Here's how the part is built. I have some questions about the finished solid (model axes, mm). A direction names the side the tool comes from. Give positions to 0.01 mm unless a question says otherwise; leave off trailing zeros. Write each loop counter-clockwise with the first axis right and the second up, starting at its lowest first coordinate (ties: lowest second). Pieces come first, ordered by that corner, then holes. Notation, with made-up numbers: (31, 41.25) - (87, 41.25) arc R33 ccw to (87, 73.25) - close; hole circle Ø7 at (70, 9). An arc over 180 degrees is marked (long way). Use one line per item in the form item = value. Start each with the question number.
from build123d import *

# Parameters (mm, degrees)
SKETCH1_W           = 158.75
SKETCH1_H           = 390.525
BOSS_EXTRUDE1_DEPTH = 3.175
SKETCH2_W           = 101.6
SKETCH2_H           = 3.175
BOSS_EXTRUDE2_DEPTH = 3.175
SKETCH3_W           = 3.175
SKETCH3_H           = 101.6
BOSS_EXTRUDE3_DEPTH = 3.175
SKETCH4_R           = 1.5875
SKETCH4_R_2         = 57.5
CUT_EXTRUDE1_DEPTH  = 426.710554544
CUT_EXTRUDE2_DEPTH  = 426.710554544
FILLET1_R           = 1.5875
FILLET2_R           = 1.5875
SKETCH7_W           = 12.7
SKETCH7_H           = 12.7
CUT_EXTRUDE3_DEPTH  = 426.710554544


with BuildPart() as part:
    # Sketch1 → Boss-Extrude1 (new body)
    with BuildSketch(Plane(origin=(0, 0, 0), x_dir=(1, 0, 0), z_dir=(0, 1, 0))):
        with Locations((79.375, 195.2625)):
            Rectangle(SKETCH1_W, SKETCH1_H)
    extrude(amount=BOSS_EXTRUDE1_DEPTH)

    # Sketch2 → Boss-Extrude2 (add)
    with BuildSketch(Plane(origin=(0, 0, 0), x_dir=(1, 0, 0), z_dir=(0, 1, 0))):
        with Locations((79.375, 392.1125)):
            Rectangle(SKETCH2_W, SKETCH2_H)
        with Locations((79.375, -1.5875)):
            Rectangle(SKETCH2_W, SKETCH2_H)
    extrude(amount=BOSS_EXTRUDE2_DEPTH)

    # Sketch3 → Boss-Extrude3 (add)
    with BuildSketch(Plane(origin=(0, 0, 0), x_dir=(1, 0, 0), z_dir=(0, 1, 0))):
        with Locations((-1.5875, 296.8625)):
            Rectangle(SKETCH3_W, SKETCH3_H)
        with Locations((-1.5875, 93.6625)):
            Rectangle(SKETCH3_W, SKETCH3_H)
        with Locations((160.3375, 93.6625)):
            Rectangle(SKETCH3_W, SKETCH3_H)
        with Locations((160.3375, 296.8625)):
            Rectangle(SKETCH3_W, SKETCH3_H)
    extrude(amount=BOSS_EXTRUDE3_DEPTH)

    # Sketch4 → Cut-Extrude1 (cut, through all)
    with BuildSketch(Plane(origin=(0, 3.175, 0), x_dir=(1, 0, 0), z_dir=(0, 1, 0))):
        with Locations(Location((26.19375, 375.4374, 0), (0, 0, 270))):
            Circle(SKETCH4_R)
        with Locations(Location((132.55625, 375.4374, 0), (0, 0, 270))):
            Circle(SKETCH4_R)
        with Locations(Location((26.19375, 269.0749, 0), (0, 0, 270))):
            Circle(SKETCH4_R)
        with Locations(Location((132.55625, 269.0749, 0), (0, 0, 270))):
            Circle(SKETCH4_R)
        with Locations(Location((79.375, 322.25615, 0), (0, 0, 270))):
            Circle(SKETCH4_R_2)
    extrude(amount=-CUT_EXTRUDE1_DEPTH, mode=Mode.SUBTRACT)

    # Sketch5 → Cut-Extrude2 (cut, through all)
    with BuildSketch(Plane(origin=(0, 3.175, 0), x_dir=(1, 0, 0), z_dir=(0, 1, 0))):
        Polygon((71.75615, 243.20615), (19.05, 190.5), (19.05, 171.45), (90.80615, 243.20615), align=None)
        Polygon((109.85615, 243.20615), (19.05, 152.4), (19.05, 133.35), (128.90615, 243.20615), align=None)
        Polygon((139.7, 234.95), (19.05, 114.3), (19.05, 95.25), (139.7, 215.9), align=None)
        Polygon((139.7, 196.85), (19.05, 76.2), (19.05, 57.15), (139.7, 177.8), align=None)
        Polygon((139.7, 158.75), (19.05, 38.1), (19.05, 19.05), (139.7, 139.7), align=None)
        Polygon((139.7, 120.65), (38.1, 19.05), (57.15, 19.05), (139.7, 101.6), align=None)
        Polygon((139.7, 82.55), (76.2, 19.05), (95.25, 19.05), (139.7, 63.5), align=None)
        Polygon((139.7, 44.45), (114.3, 19.05), (133.35, 19.05), (139.7, 25.4), align=None)
    extrude(amount=-CUT_EXTRUDE2_DEPTH, mode=Mode.SUBTRACT)

    # Fillet1
    fillet1_edges = [part.edges().sort_by_distance(p)[0] for p in [
        (0, 1.5875, -347.6625),
        (-3.175, 1.5875, -347.6625),
        (-3.175, 1.5875, -246.0625),
        (0, 1.5875, -246.0625),
        (0, 1.5875, -144.4625),
        (-3.175, 1.5875, -144.4625),
        (-3.175, 1.5875, -42.8625),
        (0, 1.5875, -42.8625),
        (0, 1.5875, 0),
        (28.575, 1.5875, 0),
        (28.575, 1.5875, 3.175),
        (130.175, 1.5875, 3.175),
        (130.175, 1.5875, 0),
        (158.75, 1.5875, 0),
        (161.925, 1.5875, -42.8625),
        (158.75, 1.5875, -42.8625),
        (161.925, 1.5875, -144.4625),
        (158.75, 1.5875, -144.4625),
        (158.75, 1.5875, -246.0625),
        (161.925, 1.5875, -246.0625),
        (161.925, 1.5875, -347.6625),
        (158.75, 1.5875, -347.6625),
        (158.75, 1.5875, -390.525),
        (130.175, 1.5875, -390.525),
        (130.175, 1.5875, -393.7),
        (28.575, 1.5875, -393.7),
        (28.575, 1.5875, -390.525),
        (0, 1.5875, -390.525),
    ]]
    fillet(fillet1_edges, radius=FILLET1_R - 0.0001)  # a hair under: the kernel refuses the full size

    # Fillet2
    fillet2_edges = [part.edges().sort_by_distance(p)[0] for p in [
        (19.05, 1.5875, -38.1),
        (139.7, 1.5875, -158.75),
        (139.7, 1.5875, -139.7),
        (19.05, 1.5875, -19.05),
        (19.05, 1.5875, -76.2),
        (139.7, 1.5875, -196.85),
        (139.7, 1.5875, -177.8),
        (19.05, 1.5875, -57.15),
        (95.25, 1.5875, -19.05),
        (76.2, 1.5875, -19.05),
        (139.7, 1.5875, -82.55),
        (139.7, 1.5875, -63.5),
        (57.15, 1.5875, -19.05),
        (38.1, 1.5875, -19.05),
        (139.7, 1.5875, -120.65),
        (139.7, 1.5875, -101.6),
        (19.05, 1.5875, -190.5),
        (71.75615, 1.5875, -243.20615),
        (90.80615, 1.5875, -243.20615),
        (19.05, 1.5875, -171.45),
        (19.05, 1.5875, -114.3),
        (139.7, 1.5875, -234.95),
        (139.7, 1.5875, -215.9),
        (19.05, 1.5875, -95.25),
        (19.05, 1.5875, -152.4),
        (109.85615, 1.5875, -243.20615),
        (128.90615, 1.5875, -243.20615),
        (19.05, 1.5875, -133.35),
        (133.35, 1.5875, -19.05),
        (114.3, 1.5875, -19.05),
        (139.7, 1.5875, -44.45),
        (139.7, 1.5875, -25.4),
    ]]
    fillet(fillet2_edges, radius=FILLET2_R)

    # Sketch7 → Cut-Extrude3 (cut, through all)
    with BuildSketch(Plane(origin=(0, 3.175, 0), x_dir=(1, 0, 0), z_dir=(0, 1, 0))):
        with Locations((25.4, 236.85615)):
            Rectangle(SKETCH7_W, SKETCH7_H)
    extrude(amount=-CUT_EXTRUDE3_DEPTH, mode=Mode.SUBTRACT)


solid = part.part
1. For P1, Ø1.6, axis at x = 140.5, y = 1.5, coming from the +Z side, with a flat end and sliding along its axis, tell me the tip position at first contact or that it passes through.
2. I want a section at C-C, the plane z = -50.5. List the corners of the cut face in (x, y) for me (3 decimals), then the cut area to 3 significant figures.
3. I want a section at A-A, the plane z = -204. List the corners of the cut face in (x, y) for me (3 decimals), then the cut area to 3 significant figures.
4. Please list where these lines run through material, in increasing order: line 1 (X direction, y = 2.1, z = -31.5); line 2 (X direction, y = 0.7, z = -135.5) (3 decimals); line 3 (X direction, y = 1, z = -175.5).
5. I want a section at B-B, the plane x = 47. Give the number of separate pieces and of enclosed holes in the cut face, then the cut area to 3 significant figures.
6. For faces 1 (the face through (60, 3.175, -198)), 2 (the face through (54.5, 1.6, -206.9)), which set-ups out of +Z, -Z, +X, -X, +Y, -Y let a thin tool reach every point of the face, with its end or its side?
7. I want a section at D-D, the plane x = 146. List the corners of the cut face in (y, z) for me (3 decimals), then the cut area to 3 significant figures.
Result sheet:
q1.P1 = 0
q2.outline = (-3.175, 0) - (31.45, 0) - (31.45, 3.175) - (-3.175, 3.175) - close; (50.5, 0) - (69.55, 0) - (69.55, 3.175) - (50.5, 3.175) - close; (88.6, 0) - (107.65, 0) - (107.65, 3.175) - (88.6, 3.175) - close; (126.7, 0) - (161.925, 0) - (161.925, 3.175) - (126.7, 3.175) - close
q2.area = 343 mm2
q3.outline = (0, 0) - (32.55, 0) - (32.55, 3.175) - (0, 3.175) - close; (51.6, 0) - (70.65, 0) - (70.65, 3.175) - (51.6, 3.175) - close; (89.7, 0) - (108.75, 0) - (108.75, 3.175) - (89.7, 3.175) - close; (127.8, 0) - (158.75, 0) - (158.75, 3.175) - (127.8, 3.175) - close
q3.area = 323 mm2
q4.line_1 = 0 to 19.05, 31.5 to 50.55, 69.6 to 88.65, 107.7 to 126.75, 139.7 to 158.75
q4.line_2 = -3.175 to 40.25, 59.3 to 78.35, 97.4 to 116.45, 135.5 to 161.925
q4.line_3 = 0 to 19.05, 23.1 to 42.15, 61.2 to 80.25, 99.3 to 118.35, 137.4 to 158.75
q5.separate_pieces = 8
q5.enclosed_holes = 0
q5.area = 628 mm2
q6.face_1 = +Z, -Z, +X, -X, +Y
q6.face_2 = +Y, -Y
q7.outline = (0, -390.525) - (3.175, -390.525) - (3.175, 0) - (0, 0) - close
q7.area = 1,240 mm2
